from build123d import *

# Parameters (mm, degrees)
BOSS_EXTRUDE2_DEPTH         = 39.6875
F_1_4_20_TAPPED_HOLE1_D     = 5.1054
F_1_4_20_TAPPED_HOLE1_DEPTH = 22.86
F_1_4_20_TAPPED_HOLE1_TIP   = 1.533816902


with BuildPart() as part:
    # Sketch3 → Boss-Extrude2 (new body, symmetric)
    with BuildSketch(Plane(origin=(0, 0, 0), x_dir=(0, 0, -1), z_dir=(1, 0, 0))):
        Polygon((0, 0), (38.1, 0), (38.1, 68.58), (0, 61.861942035), align=None)
    extrude(amount=BOSS_EXTRUDE2_DEPTH, both=True)

    # 1/4-20 Tapped Hole1
    with Locations(Plane(origin=(0, 0, 0), x_dir=(-1, 0, 0), z_dir=(0, -1, 0))):
        with Locations((25.4, 19.05), (-25.4, 19.05)):
            Hole(F_1_4_20_TAPPED_HOLE1_D / 2, depth=F_1_4_20_TAPPED_HOLE1_DEPTH)
            with Locations((0, 0, -(F_1_4_20_TAPPED_HOLE1_DEPTH + F_1_4_20_TAPPED_HOLE1_TIP / 2))):  # 118° drill point
                Cone(0, F_1_4_20_TAPPED_HOLE1_D / 2, F_1_4_20_TAPPED_HOLE1_TIP, mode=Mode.SUBTRACT)


solid = part.part
Geometry: final body of the model. Coordinates: model frame, mm. A direction names the side the tool comes from. Coordinates: 2 decimals unless noted, no trailing zeros. Loops run counter-clockwise (first coordinate to the right, second up) from the corner with the lowest first, then second, coordinate; pieces in that order, holes last. Notation, with made-up numbers: M 80.5,-0.75 L 131.5,-0.75 A10 cw 131.5,8.25 Z; hole C 59.5,-39.5 d5. An arc over 180 degrees is marked long. One line per item, written item: value. Start each with the question number.
1) Cut plane B-B (z = -32). Return loops of the section in (x, y), then the cut area to 3 significant figures.
2) Cut plane A-A (x = 13). Return loops of the section in (y, z), then the cut area to 3 significant figures.
3) Pin query (flat end, axial travel): P1, Ø4, axis at x = -25.4, z = -19.05, coming from the -Y side; P2, Ø8, axis at x = 25.4, z = -19.05, coming from the +Y side; P3, Ø3, axis at x = -15, z = -19, coming from the +Y side. Return the tip coordinate at first contact, or that it passes through.
4) Material intervals for L1, parallel to Z at x = 25.4, y = 9.25; L2, parallel to X at y = 8, z = -19.05; L3, parallel to X at y = 21, z = -18.5, sorted ascending. Write a range as from..to.
5) Draft query along Z for faces 1 (the cylindrical face through (-27.43, 11.59, -17.5)), 2 (the flat face through (1, 34, -38.1)), 3 (the flat face through (39.688, 35, -19)). Return one class per face: released by +Z, released by -Z, zero draft, split by the parting line, or undercut.
6) Reachability of faces 4 (the flat face through (1, 31, 0)), 5 (the cylindrical face through (26.578, 11.59, -16.785)) from +Z, -Z, +X, -X, +Y, -Y: full face, straight path, thin tool, end or side. Return the list, or none.
Evaluation:
1. outline: M -39.69,0 L 39.69,0 L 39.69,67.5 L -39.69,67.5 Z
1. area: 5,360 mm^2
2. outline: M 0,-38.1 L 68.58,-38.1 L 61.86,0 L 0,0 Z
2. area: 2,480 mm^2
3. P1: y = 23.19
3. P2: y = 65.93
3. P3: y = 65.48
4. L1: -38.1..-21.6, -16.5..0
4. L2: -39.69..-27.95, -22.85..22.85, 27.95..39.69
4. L3: -39.69..-27.89, -22.91..22.91, 27.89..39.69
5. face 1: undercut
5. face 2: released by -Z
5. face 3: zero draft
6. face 4: +Z, +X, -X, +Y, -Y
6. face 5: -Y
